```python
from build123d import *

# Parameters (mm, degrees)
CUT_EXTRUDE1_DEPTH = 1.3
CHAMFER1_SIZE      = 0.3


with BuildPart() as part:
    # Sketch1 → Revolve1 (revolve)
    with BuildSketch(Plane.XY):
        Polygon((0, 1.5), (8, 1.5), (8, 0), (-3, 0), (-3, 2.75), (0, 2.75), align=None)
    revolve(axis=Axis((-3, 0, 0), (1, 0, 0)))

    # Sketch2 → Cut-Revolve1 (revolve, cut)
    with BuildSketch(Plane.XY):
        Polygon((-0.948924226, 0), (-1.7, 1.25), (-3, 1.25), (-3, 0), align=None)
    revolve(axis=Axis((-3, 0, 0), (1, 0, 0)), mode=Mode.SUBTRACT)

    # Sketch3 → Cut-Extrude1 (cut)
    with BuildSketch(Plane.ZY.offset(3)):
        Polygon((1.25, 0.721687836), (0, 1.443375673), (-1.25, 0.721687836), (-1.25, -0.721687836), (0, -1.443375673), (1.25, -0.721687836), align=None)
    extrude(amount=-CUT_EXTRUDE1_DEPTH, mode=Mode.SUBTRACT)

    # Chamfer1
    chamfer1_edges = [part.edges().sort_by_distance(p)[0] for p in [
        (-3, -2.75, 0),
    ]]
    chamfer(chamfer1_edges, length=CHAMFER1_SIZE)


solid = part.part
```
Can you work these out from the model? Positions are in its coordinate system, mm. A direction names the side the tool comes from. Coordinates: 2 decimals unless noted, no trailing zeros. Loops run counter-clockwise (first coordinate to the right, second up) from the corner with the lowest first, then second, coordinate; pieces in that order, holes last. Notation, with made-up numbers: (5, 45) - (25, 45) arc R19 cw to (25, 68) - close; hole circle Ø4 at (-23, 75.5). An arc over 180 degrees is marked (long way). Use a Markdown table: item, result.
Item 1: We'd pull the mould along Z, two halves only. Please class faces 1 (the face through (0, 1.2, -1.2)), 2 (the face through (-2.36, -1.08, -0.63)), 3 (the face through (4.06, -1.5, 0.07)), 4 (the face through (-2, 0, -1.25)): released by +Z, released by -Z, zero draft, split by the parting line, or undercut.
Numbers:
| item | result |
|---|---|
| face 1 | zero draft |
| face 2 | undercut |
| face 3 | split by the parting line |
| face 4 | undercut |
Item 2: Will these pins go through, and if not, where does the flat tip stop? pin 1 (2 mm diameter, centred on x = 5, y = 0.5, fed in from +Z); pin 2 (2 mm diameter, centred on x = 2.5, z = -1.5, fed in from +Y).
Numbers:
| item | result |
|---|---|
| pin 1 | stops at z = 1.5 |
| pin 2 | stops at y = 1.41 |
Item 3: I want a section at A-A on x = -2. Please give me the cut outline in (y, z), and give its area (3 significant figures).
Numbers:
| item | result |
|---|---|
| outline | circle Ø5.5 at (0, 0); hole (-1.44, 0) - (-0.72, -1.25) - (0.72, -1.25) - (1.44, 0) - (0.72, 1.25) - (-0.72, 1.25) - close |
| area | 18.3 mm2 |
Item 4: I want a section at B-B on x = 7.5. Please give me the cut outline in (y, z), and give its area (3 significant figures).
Numbers:
| item | result |
|---|---|
| outline | circle Ø3 at (0, 0) |
| area | 7.07 mm2 |
Item 5: If I drill on probe 1 along X at (y, z) = (0.8, 1.6); probe 2 along Z at (x, y) = (3, -0.1); probe 3 along Z at (x, y) = (5.5, 0.4), over which ranges is the centre line in solid material (lowest first)? Write a range as from..to.
Numbers:
| item | result |
|---|---|
| probe 1 | x = -3..0 |
| probe 2 | z = -1.5..1.5 |
| probe 3 | z = -1.45..1.45 |
Item 6: For faces 5 (the face through (-2.36, 1.08, 0.63)), 6 (the face through (8, 0, 0)), which set-ups out of +Z, -Z, +X, -X, +Y, -Y let a thin tool reach every point of the face, with its end or its side?
Numbers:
| item | result |
|---|---|
| face 5 | -X |
| face 6 | +Z, -Z, +X, +Y, -Y |
